Can you work these out from the model? Positions are in its coordinate system, mm. A direction names the side the tool comes from. Round coordinates to 2 decimals unless told otherwise and drop trailing zeros. Order: outer loops, then holes, each group sorted by start corner. A loop starts at its lowest first (then second) coordinate and runs counter-clockwise, first axis right, second up. Notation, with made-up numbers: M 81.25,8.5 L 122.25,8.5 A10 ccw 122.25,21.5 Z; hole C 43,61 d3. An arc over 180 degrees is marked long. One line per question, with ' | ' between items.
```python
from build123d import *

# Parameters (mm, degrees)
SKETCH1_W           = 41.4
SKETCH1_H           = 24.3
BOSS_EXTRUDE1_DEPTH = 4
SKETCH2_W           = 24
SKETCH2_H           = 0.3
BOSS_EXTRUDE2_DEPTH = 3


with BuildPart() as part:
    # Sketch1 → Boss-Extrude1 (new body)
    with BuildSketch(Plane.XY):
        Rectangle(SKETCH1_W, SKETCH1_H)
    extrude(amount=-BOSS_EXTRUDE1_DEPTH)

    # Sketch2 → Boss-Extrude2 (add)
    with BuildSketch(Plane(origin=(0, 0, -4), x_dir=(-1, 0, 0), z_dir=(0, 0, -1))):
        with Locations((0, -11.55)):
            Rectangle(SKETCH2_W, SKETCH2_H)
    extrude(amount=BOSS_EXTRUDE2_DEPTH)


solid = part.part
```
(1) Will these pins go through, and if not, where does the flat tip stop? pin 1 Ø2 at (x, y) = (16.5, 9.5) entering from -Z; pin 2 Ø0.9 at (x, z) = (-6, -5.5) entering from -Y; pin 3 Ø1.5 at (x, z) = (5, -5) entering from +Y.
Final values:
pin 1: z = -4 | pin 2: y = -11.7 | pin 3: y = -11.4
(2) On a 3-axis mill with a long thin cutter (end or side, diameter ignored), from which of +Z, -Z, +X, -X, +Y, -Y can I reach the whole of each face in a straight line? I mean faces 1 (the flat face through (20.7, 0, -2)), 2 (the flat face through (0, -11.7, -5)), 3 (the flat face through (0, -11.4, -5)). Say none if no direction works.
Final values:
face 1: +Z, -Z, +X, +Y, -Y | face 2: -Z, +X, -X, -Y | face 3: -Z, +X, -X, +Y
(3) If we section it at B-B on z = -6.5: Please give me the cut outline in (x, y).
Final values:
outline: M -12,-11.7 L 12,-11.7 L 12,-11.4 L -12,-11.4 Z
(4) If we section it at C-C on y = 4: Please give me the cut outline in (x, z), plus the area to 3 significant figures.
Final values:
outline: M -20.7,-4 L 20.7,-4 L 20.7,0 L -20.7,0 Z | area: 166 mm^2
(5) If we section it at A-A on x = -8: Please give me the cut outline in (y, z), plus the area to 3 significant figures.
Final values:
outline: M -12.15,-4 L -11.7,-4 L -11.7,-7 L -11.4,-7 L -11.4,-4 L 12.15,-4 L 12.15,0 L -12.15,0 Z | area: 98.1 mm^2
(6) Please list where these lines run through material, in increasing order: probe 1 along Z at (x, y) = (17.5, 7.5); probe 2 along Y at (x, z) = (-8, -6.5). Write a range as [from, to].
Final values:
probe 1: [-4, 0] | probe 2: [-11.7, -11.4]
